```python
from build123d import *

# Parameters (mm, degrees)
BOSS_EXTRUDE1_DEPTH   = 3.175
BOSS_EXTRUDE2_DEPTH   = 3.175
F_4_CLEARANCE_HOLE1_D = 2.9464


with BuildPart() as part:
    # Sketch1 → Boss-Extrude1 (new body)
    with BuildSketch(Plane(origin=(0, 0, -14.15699402), x_dir=(-1, 0, 0), z_dir=(0, 0, -1))):
        with BuildLine():
            Line((-49.172312317, -34.502108483), (-53.141062317, -27.628031841))
            ThreePointArc((-53.141062317, -27.628031841), (-55.063803638, -24.012221257), (-56.72992661, -20.271224785))
            ThreePointArc((-56.72992661, -20.271224785), (-54.976138042, -16.13776671), (-50.842679967, -17.891555277))
            ThreePointArc((-50.842679967, -17.891555277), (-49.356678398, -21.228119699), (-47.641801003, -24.453031841))
            Line((-47.641801003, -24.453031841), (-43.673051003, -31.327108483))
            ThreePointArc((-43.673051003, -31.327108483), (-16.68272836, -52.037511462), (17.046778195, -47.596937682))
            Line((17.046778195, -47.596937682), (23.920854837, -43.628187682))
            Line((23.920854837, -43.628187682), (30.79493148, -39.659437682))
            ThreePointArc((30.79493148, -39.659437682), (51.505334458, -12.669115038), (47.064760678, 21.060391517))
            Line((47.064760678, 21.060391517), (43.096010678, 27.934468159))
            ThreePointArc((43.096010678, 27.934468159), (41.160593535, 31.032051618), (39.01404477, 33.987248938))
            ThreePointArc((39.01404477, 33.987248938), (39.561948355, 38.44382292), (44.018522337, 37.895919335))
            ThreePointArc((44.018522337, 37.895919335), (46.425258832, 34.58251628), (48.595271992, 31.109468159))
            Line((48.595271992, 31.109468159), (52.564021992, 24.235391517))
            ThreePointArc((52.564021992, 24.235391517), (57.638963455, -14.312615975), (33.96993148, -45.158698996))
            Line((33.96993148, -45.158698996), (27.095854837, -49.127448996))
            Line((27.095854837, -49.127448996), (20.221778195, -53.096198996))
            ThreePointArc((20.221778195, -53.096198996), (-18.326229296, -58.171140459), (-49.172312317, -34.502108483))
        make_face()
    extrude(amount=BOSS_EXTRUDE1_DEPTH)

    # Sketch6 → Boss-Extrude2 (add)
    with BuildSketch(Plane.XY.offset(-14.15699402)):
        Polygon((73.386475357, -62.761479903), (49.064564288, -83.169986511), (23.03238373, -52.146041808), (47.354294799, -31.7375352), align=None)
        with BuildLine():
            Line((57.786630634, -51.480655173), (60.349939064, -54.535487203))
            ThreePointArc((60.349939064, -54.535487203), (58.972420693, -70.280594225), (43.227313671, -68.903075855))
            Line((43.227313671, -68.903075855), (40.664005241, -65.848243824))
            ThreePointArc((40.664005241, -65.848243824), (42.041523612, -50.103136802), (57.786630634, -51.480655173))
        make_face(mode=Mode.SUBTRACT)
        with BuildLine():
            Line((49.261329446, -78.860212796), (46.698021016, -75.805380766))
            ThreePointArc((46.698021016, -75.805380766), (46.876472259, -73.76567372), (48.916179305, -73.944124963))
            Line((48.916179305, -73.944124963), (51.479487735, -76.998956993))
            ThreePointArc((51.479487735, -76.998956993), (51.301036492, -79.03866404), (49.261329446, -78.860212796))
        make_face(mode=Mode.SUBTRACT)
        with BuildLine():
            Line((34.124093716, -56.31560382), (36.687402146, -59.370435851))
            ThreePointArc((36.687402146, -59.370435851), (36.508950903, -61.410142897), (34.469243857, -61.231691653))
            Line((34.469243857, -61.231691653), (31.905935427, -58.176859623))
            ThreePointArc((31.905935427, -58.176859623), (32.08438667, -56.137152577), (34.124093716, -56.31560382))
        make_face(mode=Mode.SUBTRACT)
        with BuildLine():
            Line((51.752614859, -41.523518231), (54.315923289, -44.578350261))
            ThreePointArc((54.315923289, -44.578350261), (54.137472045, -46.618057308), (52.097764999, -46.439606064))
            Line((52.097764999, -46.439606064), (49.534456569, -43.384774034))
            ThreePointArc((49.534456569, -43.384774034), (49.712907813, -41.345066988), (51.752614859, -41.523518231))
        make_face(mode=Mode.SUBTRACT)
        with BuildLine():
            Line((66.544700448, -59.152039374), (69.108008878, -62.206871404))
            ThreePointArc((69.108008878, -62.206871404), (68.929557635, -64.24657845), (66.889850589, -64.068127207))
            Line((66.889850589, -64.068127207), (64.326542159, -61.013295177))
            ThreePointArc((64.326542159, -61.013295177), (64.504993402, -58.973588131), (66.544700448, -59.152039374))
        make_face(mode=Mode.SUBTRACT)
    extrude(amount=-BOSS_EXTRUDE2_DEPTH)

    # #4 Clearance Hole1 (through all)
    with Locations(Plane(origin=(0, 0, -17.33199402), x_dir=(-1, 0, 0), z_dir=(0, 0, -1))):
        with Locations((-53.56643166, -20.541270527), (-47.21643166, -31.539793155), (42.670641335, 35.021229473), (49.020641335, 24.022706845)):
            Hole(F_4_CLEARANCE_HOLE1_D / 2)


solid = part.part
```
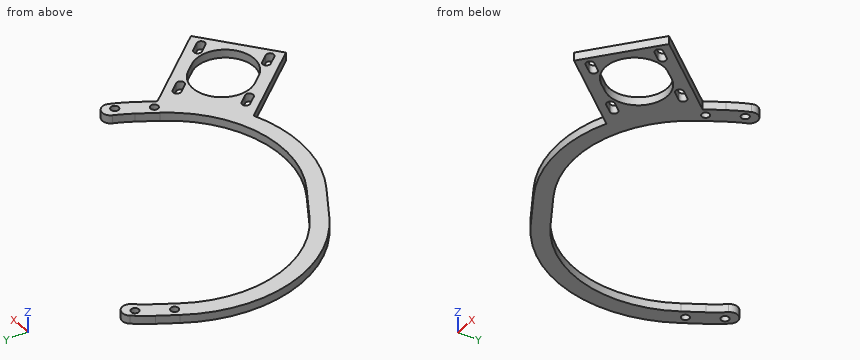
Here's how the part is built. I have some questions about the finished solid (model axes, mm). Give positions to 0.01 mm unless a question says otherwise; leave off trailing zeros. Order: outer loops, then holes, each group sorted by start corner. A loop starts at its lowest first (then second) coordinate and runs counter-clockwise, first axis right, second up. Notation, with made-up numbers: (-26.75, -11) -> (-14.75, -11) arc R20 ccw to (-14.75, 7) -> close; hole circle Ø9 at (72, -24). An arc over 180 degrees is marked (long way). Use CSV: the item, a comma, the result in double quotes. Start each with the question number.
Item 1: Suppose I cut it at C-C (x = 20). List the corners of the cut face in (y, z) for me.
Item 2: Suppose I cut it at B-B (y = 16.5). List the corners of the cut face in (x, z) for me, and give its area (3 significant figures).
Item 3: I'm going to push flat-ended pins straight in: P1, Ø2.5, axis at x = 53.57, y = -20.54, coming from the -Z side; P2, Ø1, axis at x = 13.5, z = -16.5, coming from the +Y side. Where does each tip first touch, or does it pass through?
Item 4: Suppose I cut it at A-A (z = -16.4). Give the number of separate pieces and of enclosed holes in the cut face, and give its area (3 significant figures).
Item 5: If I drill on probe 1 along X at (y, z) = (-74, -16.05); probe 2 along X at (y, z) = (-78, -14.45); probe 3 along Y at (x, z) = (-45, -15.95), over which ranges is the centre line in solid material (lowest first)? Write a range as [from, to].
Answer block:
1,outline,"(-57.69, -17.33) -> (-51.01, -17.33) -> (-51.01, -14.16) -> (-57.69, -14.16) -> close"
2,outline,"(-56.2, -17.33) -> (-49.36, -17.33) -> (-49.36, -14.16) -> (-56.2, -14.16) -> close"
2,area,"21.7 mm^2"
3,P1,"passes through"
3,P2,"stops at y = -52.67"
4,separate pieces,"1"
4,enclosed holes,"9"
4,area,"1,810 mm^2"
5,probe 1,"x = [41.37, 46.65], [48.96, 59.99]"
5,probe 2,"x = [44.73, 48.54], [51.82, 55.23]"
5,probe 3,"y = [-36.57, -26.63], [24.64, 36.6]"
